Geometry check sheet. Reference: the model listing, model coordinates, mm. A direction names the side the tool comes from. Coordinates: 2 decimals unless noted, no trailing zeros. Order: outer loops, then holes, each group sorted by start corner. A loop starts at its lowest first (then second) coordinate and runs counter-clockwise, first axis right, second up. Notation, with made-up numbers: (19.5, 46) - (74.5, 46) arc R17 ccw to (74.5, 52) - close; hole circle Ø1 at (-37.75, -27.5). An arc over 180 degrees is marked (long way). Use CSV: the item, a comma, the result in double quotes. Start each with the question number.
1) Sectioned sample at B-B, the plane z = -7.5. Count the separate pieces of the cut face and the enclosed holes in it, and give its area (3 significant figures).
2) Draft check along Z on faces 4 (the flat face through (16.075, 3, -6)), 5 (the cylindrical face through (-0.65, 1.48, -5.93)), 6 (the flat face through (0, 2, -12)). Enter one of: released by +Z, released by -Z, zero draft, split by the parting line, or undercut.
3) Sectioned sample at D-D, the plane x = -10. Record the cut outline in (y, z) (3 decimals), and give its area (3 significant figures).
4) Tool access check on faces 1 (the flat face through (-3.925, 2, -6)), 2 (the conical face through (-9.863, 4.635, 6.209)), 3 (the cylindrical face through (-10.186, 0.197, 8.473)). Record the directions out of +Z, -Z, +X, -X, +Y, -Y that give a thin tool (end or side, any length) a straight path to the whole face; none if there is none.
5) Sectioned sample at C-C, the plane x = 10. Record the cut outline in (y, z) (3 decimals).
6) Thickness scan on probe 1 along X at (y, z) = (0.9, -7.5) (3 decimals); probe 2 along X at (y, z) = (1.7, -9.25) (3 decimals); probe 3 along X at (y, z) = (1, -0.5) (3 decimals). Record the ranges inside material, lowest first. Write a range as [from, to].
7) Sectioned sample at A-A, the plane x = 0. Record the cut outline in (y, z).
from build123d import *

# Parameters (mm, degrees)
SKETCH1_R           = 1.7
SKETCH1_R_2         = 2.5
BOSS_EXTRUDE1_DEPTH = 5
CHAMFER2_SIZE       = 2
CUT_EXTRUDE1_DEPTH  = 0.4
CHAMFER1_SIZE       = 0.5


with BuildPart() as part:
    # Sketch1 → Boss-Extrude1 (new body)
    with BuildSketch(Plane(origin=(0, 0, 0), x_dir=(1, 0, 0), z_dir=(0, 1, 0))):
        with BuildLine():
            Line((-35, -12), (35, -12))
            Line((35, -12), (35, 12))
            Line((35, 12), (16.075, 12))
            Line((16.075, 12), (16.075, 0))
            ThreePointArc((16.075, 0), (10, -6.075), (3.925, 0))
            Line((3.925, 0), (3.925, 12))
            Line((3.925, 12), (-3.925, 12))
            Line((-3.925, 12), (-3.925, 0))
            ThreePointArc((-3.925, 0), (-10, -6.075), (-16.075, 0))
            Line((-16.075, 0), (-16.075, 12))
            Line((-16.075, 12), (-35, 12))
            Line((-35, 12), (-35, -12))
        make_face()
        with Locations(Location((0, -7.5, 0), (0, 0, 270))):
            Circle(SKETCH1_R, mode=Mode.SUBTRACT)
        with Locations(Location((-24.875, 0, 0), (0, 0, 270))):
            Circle(SKETCH1_R_2, mode=Mode.SUBTRACT)
        with Locations(Location((24.875, 0, 0), (0, 0, 270))):
            Circle(SKETCH1_R_2, mode=Mode.SUBTRACT)
        with Locations(Location((0, 7.5, 0), (0, 0, 270))):
            Circle(SKETCH1_R, mode=Mode.SUBTRACT)
    extrude(amount=BOSS_EXTRUDE1_DEPTH)

    # Chamfer2
    chamfer2_edges = [part.edges().sort_by_distance(p)[0] for p in [
        (0, 5, 5.8),
        (0, 5, -9.2),
    ]]
    chamfer(chamfer2_edges, length=CHAMFER2_SIZE)

    # Sketch2 → Cut-Extrude1 (cut)
    with BuildSketch(Plane.XZ):
        with BuildLine():
            Line((-1.525, 0), (-1.525, -12))
            Line((-1.525, -12), (-18.475, -12))
            Line((-18.475, -12), (-18.475, 0))
            ThreePointArc((-18.475, 0), (-10, 8.475), (-1.525, 0))
        make_face()
        with BuildLine():
            Line((18.475, -12), (1.525, -12))
            Line((1.525, -12), (1.525, 0))
            ThreePointArc((1.525, 0), (10, 8.475), (18.475, 0))
            Line((18.475, 0), (18.475, -12))
        make_face()
    extrude(amount=-CUT_EXTRUDE1_DEPTH, mode=Mode.SUBTRACT)

    # Chamfer1
    chamfer1_edges = [part.edges().sort_by_distance(p)[0] for p in [
        (0, 0, 12),
    ]]
    chamfer(chamfer1_edges, length=CHAMFER1_SIZE)
    chamfer1_2_edges = [part.edges().sort_by_distance(p)[0] for p in [
        (0, 5, 12),
    ]]
    chamfer(chamfer1_2_edges, length=CHAMFER1_SIZE)
    chamfer1_3_edges = [part.edges().sort_by_distance(p)[0] for p in [
        (16.075, 0.4, -6),
        (10, 0.4, 6.075),
        (3.925, 0.4, -6),
    ]]
    chamfer(chamfer1_3_edges, length=CHAMFER1_SIZE)
    chamfer1_4_edges = [part.edges().sort_by_distance(p)[0] for p in [
        (35, 0, -0.25),
    ]]
    chamfer(chamfer1_4_edges, length=CHAMFER1_SIZE)
    chamfer1_5_edges = [part.edges().sort_by_distance(p)[0] for p in [
        (-35, 0, -0.25),
    ]]
    chamfer(chamfer1_5_edges, length=CHAMFER1_SIZE)
    chamfer1_6_edges = [part.edges().sort_by_distance(p)[0] for p in [
        (-35, 5, -0.25),
    ]]
    chamfer(chamfer1_6_edges, length=CHAMFER1_SIZE)
    chamfer1_7_edges = [part.edges().sort_by_distance(p)[0] for p in [
        (35, 5, -0.25),
    ]]
    chamfer(chamfer1_7_edges, length=CHAMFER1_SIZE)
    chamfer1_8_edges = [part.edges().sort_by_distance(p)[0] for p in [
        (25.2875, 5, -12),
    ]]
    chamfer(chamfer1_8_edges, length=CHAMFER1_SIZE)
    chamfer1_9_edges = [part.edges().sort_by_distance(p)[0] for p in [
        (-25.2875, 5, -12),
    ]]
    chamfer(chamfer1_9_edges, length=CHAMFER1_SIZE)
    chamfer1_10_edges = [part.edges().sort_by_distance(p)[0] for p in [
        (26.4875, 0, -12),
    ]]
    chamfer(chamfer1_10_edges, length=CHAMFER1_SIZE)
    chamfer1_11_edges = [part.edges().sort_by_distance(p)[0] for p in [
        (-26.4875, 0, -12),
    ]]
    chamfer(chamfer1_11_edges, length=CHAMFER1_SIZE)
    chamfer1_12_edges = [part.edges().sort_by_distance(p)[0] for p in [
        (0, 5, -12),
    ]]
    chamfer(chamfer1_12_edges, length=CHAMFER1_SIZE)
    chamfer1_13_edges = [part.edges().sort_by_distance(p)[0] for p in [
        (0, 0, -12),
    ]]
    chamfer(chamfer1_13_edges, length=CHAMFER1_SIZE)
    # the kernel refuses this chamfer: 0.5 mm, written as the material it takes off along each edge
    with BuildSketch(Plane(origin=(16.075, 5, -12.785841494), x_dir=(0.9996219169112968, 0.02749587661058555, 0), z_dir=(0, 0, 1)), Plane(origin=(3.925, 5, 0), x_dir=(-0.9996219169112968, 0.027495876610585623, 0), z_dir=(0, 0, -1))) as chamfer1_14_piece_1:
        with BuildLine():
            Line((0.514336598, 0), (-0.028273577, -0.513558897))
            Line((-0.028273577, -0.513558897), (-0.038269797, -0.513283938))
            ThreePointArc((-0.038269797, -0.513283938), (-0.017064614, -0.256698915), (-0.009996219, 0.000274959))
            Line((-0.009996219, 0.000274959), (0.000274959, 0.009996219))
            ThreePointArc((0.000274959, 0.009996219), (0.257248832, 0.002927825), (0.514611556, 0.009996219))
            Line((0.514611556, 0.009996219), (0.514336598, 0))
        make_face()
    extrude(amount=12.785841494, mode=Mode.SUBTRACT)
    with BuildSketch(Plane(origin=(10, 5, 0), x_dir=(1, 0, 0), z_dir=(0, 0, -1))) as chamfer1_14_piece_2:
        with BuildLine():
            Line((6.589142136, -0.014142136), (6.060857864, 0.514142136))
            Line((6.060857864, 0.514142136), (6.050857864, 0.514142136))
            ThreePointArc((6.050857864, 0.514142136), (6.065, 0.257071068), (6.065, 0))
            Line((6.065, 0), (6.075, -0.01))
            ThreePointArc((6.075, -0.01), (6.332071068, -0.01), (6.589142136, -0.024142136))
            Line((6.589142136, -0.024142136), (6.589142136, -0.014142136))
        make_face()
    revolve(axis=Axis((10, 5, 0), (0, -1, 0)), revolution_arc=180, mode=Mode.SUBTRACT)
    # the kernel refuses this chamfer: 0.5 mm, written as the material it takes off along each edge
    with BuildSketch(Plane(origin=(-3.925, 5, -12.785841494), x_dir=(-0.02749587661058651, -0.9996219169112968, 0), z_dir=(0, 0, 1))) as chamfer1_15_piece_1:
        with BuildLine():
            Line((0.514336598, 0), (-0.028273577, 0.513558897))
            Line((-0.028273577, 0.513558897), (-0.038269797, 0.513283938))
            ThreePointArc((-0.038269797, 0.513283938), (-0.017064614, 0.256698915), (-0.009996219, -0.000274959))
            Line((-0.009996219, -0.000274959), (0.000274959, -0.009996219))
            ThreePointArc((0.000274959, -0.009996219), (0.257248832, -0.002927825), (0.514611556, -0.009996219))
            Line((0.514611556, -0.009996219), (0.514336598, 0))
        make_face()
    extrude(amount=12.785841494, mode=Mode.SUBTRACT)
    with BuildSketch(Plane(origin=(-10, 5, 0), x_dir=(1, 0, 0), z_dir=(0, 0, -1))) as chamfer1_15_piece_2:
        with BuildLine():
            Line((6.589142136, -0.014142136), (6.060857864, 0.514142136))
            Line((6.060857864, 0.514142136), (6.050857864, 0.514142136))
            ThreePointArc((6.050857864, 0.514142136), (6.065, 0.257071068), (6.065, 0))
            Line((6.065, 0), (6.075, -0.01))
            ThreePointArc((6.075, -0.01), (6.332071068, -0.01), (6.589142136, -0.024142136))
            Line((6.589142136, -0.024142136), (6.589142136, -0.014142136))
        make_face()
    revolve(axis=Axis((-10, 5, 0), (0, -1, 0)), revolution_arc=180, mode=Mode.SUBTRACT)
    with BuildSketch(Plane(origin=(-16.075, 5, 0), x_dir=(-0.9996219169112968, 0.02749587661058555, 0), z_dir=(0, 0, -1))) as chamfer1_15_piece_3:
        with BuildLine():
            Line((0.514336598, 0), (-0.028273577, -0.513558897))
            Line((-0.028273577, -0.513558897), (-0.038269797, -0.513283938))
            ThreePointArc((-0.038269797, -0.513283938), (-0.017064614, -0.256698915), (-0.009996219, 0.000274959))
            Line((-0.009996219, 0.000274959), (0.000274959, 0.009996219))
            ThreePointArc((0.000274959, 0.009996219), (0.257248832, 0.002927825), (0.514611556, 0.009996219))
            Line((0.514611556, 0.009996219), (0.514336598, 0))
        make_face()
    extrude(amount=12.785841494, mode=Mode.SUBTRACT)


solid = part.part
Evaluation:
1,separate pieces,"4"
1,enclosed holes,"0"
1,area,"203 mm²"
2,face 4,"zero draft"
2,face 5,"undercut"
2,face 6,"released by -Z"
3,outline,"(0, 8.475) - (0.4, 8.475) - (0.4, 6.075) - (4.5, 6.075) - (5, 6.575) - (5, 11.5) - (4.5, 12) - (0.5, 12) - (0, 11.5) - close"
3,area,"28.3 mm²"
4,face 1,"-Z, +Y, -Y"
4,face 2,"-Z, +Y"
4,face 3,"-Z, -Y"
5,outline,"(0, 8.475) - (0.4, 8.475) - (0.4, 6.575) - (0.9, 6.075) - (4.5, 6.075) - (5, 6.575) - (5, 11.5) - (4.5, 12) - (0.5, 12) - (0, 11.5) - close"
6,probe 1,"[-35, -16.075], [-3.925, -1.7], [1.7, 3.925], [16.075, 35]"
6,probe 2,"[-35, -16.075], [-3.925, 3.925], [16.075, 35]"
6,probe 3,"[-35, -27.324], [-22.426, -16.075], [-3.925, 3.925], [16.075, 22.426], [27.324, 35]"
7,outline,"(0, -11.5) - (0.5, -12) - (4.5, -12) - (5, -11.5) - (5, -11.2) - (3, -9.2) - (0, -9.2) - close; (0, -5.8) - (3, -5.8) - (5, -3.8) - (5, 3.8) - (3, 5.8) - (0, 5.8) - close; (0, 9.2) - (3, 9.2) - (5, 11.2) - (5, 11.5) - (4.5, 12) - (0.5, 12) - (0, 11.5) - close"
